Study the drawing (mm; zero at the part's minimum x, y, z) and answer. A direction names the side the tool comes from. Coordinates: 2 decimals unless noted, no trailing zeros. Loops run counter-clockwise (first coordinate to the right, second up) from the corner with the lowest first, then second, coordinate; pieces in that order, holes last.
Q1. The mould has two halves that part along Z. Classify the marked faces 3, 4, 5 and 6: pulls with the +Z half, pulls with the -Z half, needs draft (parallel to the pull), parting line crosses it, or undercut.
Q2. Straight lines are drawn through the part: line 1 (Z direction, x = 33, y = 3.7); line 2 (X direction, y = 6, z = 9.5); line 3 (X direction, y = 6.75, z = 8.5). For each, find the intervals that lie inside material, in ascending order.
Q3. Section D-D (x = 24) is taken. Give the vertices of the cut face in (y, z).
Q4. Flat-ended cylindrical pins translate along their axes: P1, Ø3.5, axis at x = 33, z = 10, coming from the +Y side; P2, Ø4.5, axis at x = 7, z = 10, coming from the -Y side. Find the tip coordinate at first contact, or state that the pin passes through.
Q5. Which of the six approach directions +Z, -Z, +X, -X, +Y, -Y give full straight-line access (tool end or side, diameter ignored) to the marked faces 1 and 2?
Q6. Section A-A (z = 10) is taken. Give the vertices of the cut face in (x, y), then the cut area to 3 significant figures.
Q7. Section B-B (y = 1) is taken. Give the vertices of the cut face in (x, z), then the cut area to 3 significant figures.
Q8. Section C-C (x = 33) is taken. Give the vertices of the cut face in (y, z).
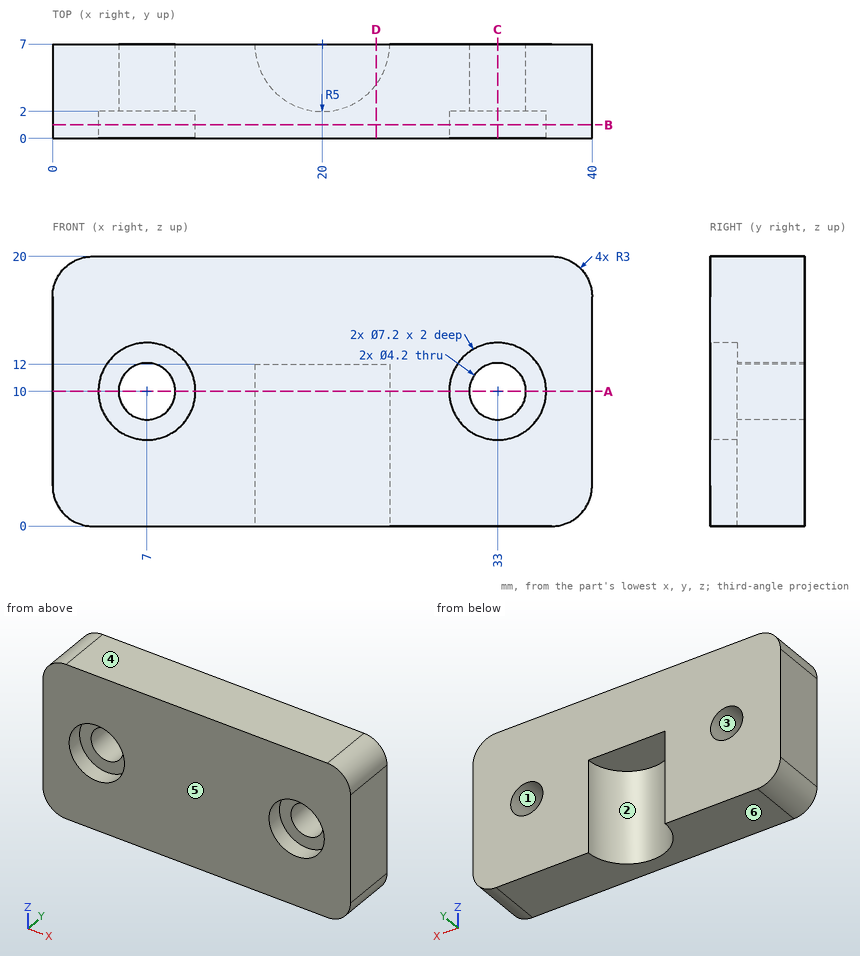
Numbers:
1. face 3: undercut
1. face 4: pulls with the +Z half
1. face 5: needs draft
1. face 6: pulls with the -Z half
2. line 1: z = 0 to 7.9, 12.1 to 20
2. line 2: x = 0 to 4.96, 9.04 to 15.1, 24.9 to 30.96, 35.04 to 40
2. line 3: x = 0 to 5.53, 8.47 to 15.01, 24.99 to 31.53, 34.47 to 40
3. outline: (0, 0) - (4, 0) - (4, 12) - (7, 12) - (7, 20) - (0, 20) - close
4. P1: passes through
4. P2: stops at y = 2
5. face 1: +Y, -Y
5. face 2: -Z, +Y
6. outline: (0, 0) - (3.4, 0) - (3.4, 2) - (4.9, 2) - (4.9, 7) - (0, 7) - close; (9.1, 2) - (10.6, 2) - (10.6, 0) - (29.4, 0) - (29.4, 2) - (30.9, 2) - (30.9, 7) - (25, 7) arc R5 cw to (15, 7) - (9.1, 7) - close; (35.1, 2) - (36.6, 2) - (36.6, 0) - (40, 0) - (40, 7) - (35.1, 7) - close
6. area: 170 mm2
7. outline: (0, 3) arc R3 ccw to (3, 0) - (37, 0) arc R3 ccw to (40, 3) - (40, 17) arc R3 ccw to (37, 20) - (3, 20) arc R3 ccw to (0, 17) - close; hole circle Ø7.2 at (7, 10); hole circle Ø7.2 at (33, 10)
7. area: 711 mm2
8. outline: (0, 0) - (7, 0) - (7, 7.9) - (2, 7.9) - (2, 6.4) - (0, 6.4) - close; (0, 13.6) - (2, 13.6) - (2, 12.1) - (7, 12.1) - (7, 20) - (0, 20) - close
